Part model, mm, in its own coordinate system. A direction names the side the tool comes from. Round coordinates to 2 decimals unless told otherwise and drop trailing zeros. Loops run counter-clockwise (first coordinate to the right, second up) from the corner with the lowest first, then second, coordinate; pieces in that order, holes last.
from build123d import *

# Parameters (mm, degrees)
SKETCH_1_W            = 114
SKETCH_1_H            = 62
EXTRUDE_1_DEPTH       = 5.6
SKETCH_5_R            = 3
CUT_EXTRUDE_865_DEPTH = 3
SKETCH_7_W            = 85
SKETCH_7_H            = 58
LCD_DEPTH             = 3.6
SKETCH_13_W           = 74
SKETCH_13_H           = 46
CUT_EXTRUDE_1_DEPTH   = 10
FILLET_2_R            = 5
FILLET_3_R            = 6


with BuildPart() as part:
    # Эскиз1 → Бобышка-Вытянуть1 (new body)
    with BuildSketch(Plane(origin=(0, 0, 0), x_dir=(1, 0, 0), z_dir=(0, 1, 0))):
        with Locations((-2, 0)):
            Rectangle(SKETCH_1_W, SKETCH_1_H)
    extrude(amount=EXTRUDE_1_DEPTH)

    # Эскиз5 → Cut-Extrude 865 (cut)
    with BuildSketch(Plane.XZ):
        with Locations(Location((-54, 21, 0), (0, 0, 270))):
            Circle(SKETCH_5_R)
        with Locations(Location((-54, -21, 0), (0, 0, 90))):
            Circle(SKETCH_5_R)
        with Locations(Location((39, 21, 0), (0, 0, 270))):
            Circle(SKETCH_5_R)
        with Locations(Location((39, -21, 0), (0, 0, 90))):
            Circle(SKETCH_5_R)
    extrude(amount=-CUT_EXTRUDE_865_DEPTH, mode=Mode.SUBTRACT)

    # Эскиз7 → под LCD (cut)
    with BuildSketch(Plane.XZ):
        with Locations((-7.5, 0)):
            Rectangle(SKETCH_7_W, SKETCH_7_H)
    extrude(amount=-LCD_DEPTH, mode=Mode.SUBTRACT)

    # Эскиз13 → Вырез-Вытянуть1 (cut)
    with BuildSketch(Plane.XZ.offset(-3.6)):
        with Locations((-6, 0)):
            Rectangle(SKETCH_13_W, SKETCH_13_H)
    extrude(amount=-CUT_EXTRUDE_1_DEPTH, mode=Mode.SUBTRACT)

    # Скругление2
    # the kernel refuses this fillet: 5 mm, written as the material it takes off along each edge
    with BuildSketch(Plane(origin=(-43, 5.6, 23), x_dir=(-1, 0, 0), z_dir=(0, 0, -1)), Plane(origin=(31, 5.6, -23), x_dir=(1, 0, 0), z_dir=(0, 0, 1))) as fillet_2_piece_1:
        with BuildLine():
            CenterArc((4, -5), FILLET_2_R, 90, 53.130102354)
            Line((0, -2), (-0.08, -1.94))
            ThreePointArc((-0.08, -1.94), (-0.1, -1), (-0.1, 0))
            Line((-0.1, 0), (0, 0.1))
            Line((0, 0.1), (4, 0.1))
            Line((4, 0.1), (4, 0))
        make_face()
    extrude(amount=46, mode=Mode.SUBTRACT)
    with BuildSketch(Plane(origin=(31, 5.6, 23), x_dir=(0, 0, 1), z_dir=(-1, 0, 0)), Plane(origin=(-43, 5.6, -23), x_dir=(0, 0, -1), z_dir=(1, 0, 0))) as fillet_2_piece_2:
        with BuildLine():
            CenterArc((4, -5), FILLET_2_R, 90, 53.130102354)
            Line((0, -2), (-0.08, -1.94))
            ThreePointArc((-0.08, -1.94), (-0.1, -1), (-0.1, 0))
            Line((-0.1, 0), (0, 0.1))
            Line((0, 0.1), (4, 0.1))
            Line((4, 0.1), (4, 0))
        make_face()
    extrude(amount=74, mode=Mode.SUBTRACT)
    with BuildSketch(Plane(origin=(31, 5.6, 23), x_dir=(0, 0, 1), z_dir=(-1, 0, 0))) as fillet_2_piece_3a_section:
        with BuildLine():
            CenterArc((4, -5), FILLET_2_R, 90, 53.130102354)
            Line((0, -2), (-0.08, -1.94))
            ThreePointArc((-0.08, -1.94), (-0.1, -1), (-0.1, 0))
            Line((-0.1, 0), (0, 0.1))
            Line((0, 0.1), (4, 0.1))
            Line((4, 0.1), (4, 0))
        make_face()
    fillet_2_piece_3a = extrude(amount=84, mode=Mode.PRIVATE)
    fillet_2_piece_3a = split(fillet_2_piece_3a, bisect_by=Plane(origin=(-43, 5.088057438, 24.029417057), z_dir=(-1, 0, 0)), keep=Keep.TOP, mode=Mode.PRIVATE)
    with BuildSketch(Plane(origin=(-43, 5.6, 33), x_dir=(-1, 0, 0), z_dir=(0, 0, -1))) as fillet_2_piece_3b_section:
        with BuildLine():
            CenterArc((4, -5), FILLET_2_R, 90, 53.130102354)
            Line((0, -2), (-0.08, -1.94))
            ThreePointArc((-0.08, -1.94), (-0.1, -1), (-0.1, 0))
            Line((-0.1, 0), (0, 0.1))
            Line((0, 0.1), (4, 0.1))
            Line((4, 0.1), (4, 0))
        make_face()
    fillet_2_piece_3b = extrude(amount=56, mode=Mode.PRIVATE)
    fillet_2_piece_3b = split(fillet_2_piece_3b, bisect_by=Plane(origin=(-44.029417057, 5.088057438, 23), z_dir=(0, 0, 1)), keep=Keep.TOP, mode=Mode.PRIVATE)
    fillet_2_piece_3 = fillet_2_piece_3a & fillet_2_piece_3b
    add(fillet_2_piece_3, mode=Mode.SUBTRACT)
    with BuildSketch(Plane(origin=(-43, 5.6, 23), x_dir=(-1, 0, 0), z_dir=(0, 0, -1))) as fillet_2_piece_4a_section:
        with BuildLine():
            CenterArc((4, -5), FILLET_2_R, 90, 53.130102354)
            Line((0, -2), (-0.08, -1.94))
            ThreePointArc((-0.08, -1.94), (-0.1, -1), (-0.1, 0))
            Line((-0.1, 0), (0, 0.1))
            Line((0, 0.1), (4, 0.1))
            Line((4, 0.1), (4, 0))
        make_face()
    fillet_2_piece_4a = extrude(amount=56, mode=Mode.PRIVATE)
    fillet_2_piece_4a = split(fillet_2_piece_4a, bisect_by=Plane(origin=(-44.029417057, 5.088057438, -23), z_dir=(0, 0, -1)), keep=Keep.TOP, mode=Mode.PRIVATE)
    with BuildSketch(Plane(origin=(-53, 5.6, -23), x_dir=(0, 0, -1), z_dir=(1, 0, 0))) as fillet_2_piece_4b_section:
        with BuildLine():
            CenterArc((4, -5), FILLET_2_R, 90, 53.130102354)
            Line((0, -2), (-0.08, -1.94))
            ThreePointArc((-0.08, -1.94), (-0.1, -1), (-0.1, 0))
            Line((-0.1, 0), (0, 0.1))
            Line((0, 0.1), (4, 0.1))
            Line((4, 0.1), (4, 0))
        make_face()
    fillet_2_piece_4b = extrude(amount=84, mode=Mode.PRIVATE)
    fillet_2_piece_4b = split(fillet_2_piece_4b, bisect_by=Plane(origin=(-43, 5.088057438, -24.029417057), z_dir=(-1, 0, 0)), keep=Keep.TOP, mode=Mode.PRIVATE)
    fillet_2_piece_4 = fillet_2_piece_4a & fillet_2_piece_4b
    add(fillet_2_piece_4, mode=Mode.SUBTRACT)
    with BuildSketch(Plane(origin=(41, 5.6, 23), x_dir=(0, 0, 1), z_dir=(-1, 0, 0))) as fillet_2_piece_5a_section:
        with BuildLine():
            CenterArc((4, -5), FILLET_2_R, 90, 53.130102354)
            Line((0, -2), (-0.08, -1.94))
            ThreePointArc((-0.08, -1.94), (-0.1, -1), (-0.1, 0))
            Line((-0.1, 0), (0, 0.1))
            Line((0, 0.1), (4, 0.1))
            Line((4, 0.1), (4, 0))
        make_face()
    fillet_2_piece_5a = extrude(amount=84, mode=Mode.PRIVATE)
    fillet_2_piece_5a = split(fillet_2_piece_5a, bisect_by=Plane(origin=(31, 5.088057438, 24.029417057), z_dir=(1, 0, 0)), keep=Keep.TOP, mode=Mode.PRIVATE)
    with BuildSketch(Plane(origin=(31, 5.6, -23), x_dir=(1, 0, 0), z_dir=(0, 0, 1))) as fillet_2_piece_5b_section:
        with BuildLine():
            CenterArc((4, -5), FILLET_2_R, 90, 53.130102354)
            Line((0, -2), (-0.08, -1.94))
            ThreePointArc((-0.08, -1.94), (-0.1, -1), (-0.1, 0))
            Line((-0.1, 0), (0, 0.1))
            Line((0, 0.1), (4, 0.1))
            Line((4, 0.1), (4, 0))
        make_face()
    fillet_2_piece_5b = extrude(amount=56, mode=Mode.PRIVATE)
    fillet_2_piece_5b = split(fillet_2_piece_5b, bisect_by=Plane(origin=(32.029417057, 5.088057438, 23), z_dir=(0, 0, 1)), keep=Keep.TOP, mode=Mode.PRIVATE)
    fillet_2_piece_5 = fillet_2_piece_5a & fillet_2_piece_5b
    add(fillet_2_piece_5, mode=Mode.SUBTRACT)
    with BuildSketch(Plane(origin=(-43, 5.6, -23), x_dir=(0, 0, -1), z_dir=(1, 0, 0))) as fillet_2_piece_6a_section:
        with BuildLine():
            CenterArc((4, -5), FILLET_2_R, 90, 53.130102354)
            Line((0, -2), (-0.08, -1.94))
            ThreePointArc((-0.08, -1.94), (-0.1, -1), (-0.1, 0))
            Line((-0.1, 0), (0, 0.1))
            Line((0, 0.1), (4, 0.1))
            Line((4, 0.1), (4, 0))
        make_face()
    fillet_2_piece_6a = extrude(amount=84, mode=Mode.PRIVATE)
    fillet_2_piece_6a = split(fillet_2_piece_6a, bisect_by=Plane(origin=(31, 5.088057438, -24.029417057), z_dir=(1, 0, 0)), keep=Keep.TOP, mode=Mode.PRIVATE)
    with BuildSketch(Plane(origin=(31, 5.6, -33), x_dir=(1, 0, 0), z_dir=(0, 0, 1))) as fillet_2_piece_6b_section:
        with BuildLine():
            CenterArc((4, -5), FILLET_2_R, 90, 53.130102354)
            Line((0, -2), (-0.08, -1.94))
            ThreePointArc((-0.08, -1.94), (-0.1, -1), (-0.1, 0))
            Line((-0.1, 0), (0, 0.1))
            Line((0, 0.1), (4, 0.1))
            Line((4, 0.1), (4, 0))
        make_face()
    fillet_2_piece_6b = extrude(amount=56, mode=Mode.PRIVATE)
    fillet_2_piece_6b = split(fillet_2_piece_6b, bisect_by=Plane(origin=(32.029417057, 5.088057438, -23), z_dir=(0, 0, -1)), keep=Keep.TOP, mode=Mode.PRIVATE)
    fillet_2_piece_6 = fillet_2_piece_6a & fillet_2_piece_6b
    add(fillet_2_piece_6, mode=Mode.SUBTRACT)

    # Скругление3
    fillet_3_edges = [part.edges().sort_by_distance(p)[0] for p in [
        (55, 2.8, 31),
        (-59, 2.8, 31),
        (-59, 2.8, -31),
        (55, 2.8, -31),
    ]]
    fillet(fillet_3_edges, radius=FILLET_3_R)


solid = part.part
1) Slice it at C-C, the plane y = 1.9. Give the cut face in (x, z), then the cut area to 3 significant figures.
Values:
outline: (-59, -25) arc R6 ccw to (-53, -31) - (49, -31) arc R6 ccw to (55, -25) - (55, 25) arc R6 ccw to (49, 31) - (-53, 31) arc R6 ccw to (-59, 25) - close; hole circle Ø6 at (-54, -21); hole circle Ø6 at (-54, 21); hole (-50, -29) - (35, -29) - (35, 29) - (-50, 29) - close; hole circle Ø6 at (39, -21); hole circle Ø6 at (39, 21)
area: 1,990 mm2
2) Slice it at D-D, the plane z = -21. Give the cut face in (x, y), then the cut area to 3 significant figures.
Values:
outline: (-59, 0) - (-57, 0) - (-57, 3) - (-51, 3) - (-51, 0) - (-50, 0) - (-50, 3.6) - (-43, 3.6) arc R5 ccw to (-47, 5.6) - (-59, 5.6) - close; (31, 3.6) - (35, 3.6) - (35, 0) - (36, 0) - (36, 3) - (42, 3) - (42, 0) - (55, 0) - (55, 5.6) - (35, 5.6) arc R5 ccw to start
area: 144 mm2
3) Slice it at A-A, the plane z = 12.5. Give the cut face in (x, y).
Values:
outline: (-59, 0) - (-50, 0) - (-50, 3.6) - (-43, 3.6) arc R5 ccw to (-47, 5.6) - (-59, 5.6) - close; (31, 3.6) - (35, 3.6) - (35, 0) - (55, 0) - (55, 5.6) - (35, 5.6) arc R5 ccw to start
4) Wall check: line 1 along X through (y, z) = (1.35, 21); line 2 along X through (y, z) = (1.9, -25.5); line 3 along Z through (x, y) = (31, 1.6). Give the ranges that are in metal, low to high.
Values:
line 1: x = -59 to -57, -51 to -50, 35 to 36, 42 to 55
line 2: x = -58.98 to -50, 35 to 54.98
line 3: z = -31 to -29, 29 to 31
5) Mould opens along Z. For faces 4 (the face through (53.289, 2.839, 29.196)), 5 (the face through (-59, 3, 0)), 6 (the face through (-57, 1, -21)) say: released by +Z, released by -Z, zero draft, split by the parting line, or undercut.
Values:
face 4: released by +Z
face 5: zero draft
face 6: undercut
6) Tool access for faces 1 (the face through (32.793, 5.087, -0.378)), 2 (the face through (-14, 3.6, -23.5)), 3 (the face through (-57.289, 2.839, -29.196)): list every direction of +Z, -Z, +X, -X, +Y, -Y with a clear straight run to the whole face (end or side of a thin tool).
Values:
face 1: +Y
face 2: -Y
face 3: -Z, -X, +Y, -Y
7) Slice it at B-B, the plane x = 9. Give the cut face in (y, z).
Values:
outline: (0, -31) - (5.6, -31) - (5.6, -27) arc R5 ccw to (3.6, -23) - (3.6, -29) - (0, -29) - close; (0, 29) - (3.6, 29) - (3.6, 23) arc R5 ccw to (5.6, 27) - (5.6, 31) - (0, 31) - close
8) Drop flat-ended pins along their axis: pin 1 Ø5 at (x, z) = (40.5, 21) entering from -Y; pin 2 Ø1.8 at (x, z) = (-55, 22) entering from -Y. Give the stop position or say it passes through.
Values:
pin 1: stops at y = 0
pin 2: stops at y = 3
